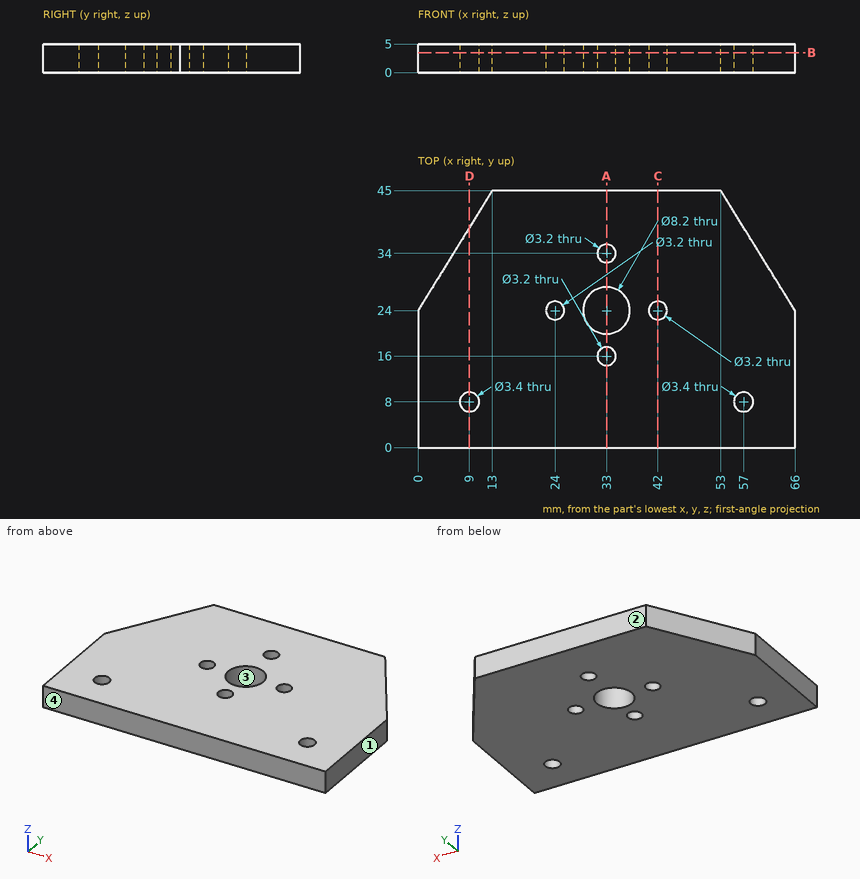
Study the drawing (mm; zero at the part's minimum x, y, z) and answer. Coordinates: 2 decimals unless noted, no trailing zeros. Loops run counter-clockwise (first coordinate to the right, second up) from the corner with the lowest first, then second, coordinate; pieces in that order, holes last. Notation, with made-up numbers: M 48.5,74.5 L 84.5,74.5 A24 cw 84.5,93.5 Z; hole C 60.5,-33 d3. An arc over 180 degrees is marked long. Answer as a JSON object with one key per item and string values. Group by question number.
Item 1: Section A-A (x = 33) is taken. Write down the section's boundary in (y, z).
Item 2: Section D-D (x = 9) is taken. Write down the section's boundary in (y, z).
Item 3: Section C-C (x = 42) is taken. Write down the section's boundary in (y, z).
Item 4: Consider L1, parallel to Y at x = 33, z = 3.55; L2, parallel to X at y = 26.5, z = 3.35; L3, parallel to X at y = 15.5, z = 2.7. Determine where each line is inside the solid, lowest interval first.
Item 5: Determine the mould class of the marked faces 1, 2, 3 and 4 for opening direction Y: +Y half, -Y half, draft (parallel to the pull), parting line (faces both ways), or undercut.
Item 6: Section B-B (z = 3.5) is taken. Write down the section's boundary in (x, y).
Item 7: Each of these flat-tipped pins is pushed along its axis until it touches: P1, Ø3, axis at y = 32.5, z = 3, coming from the +X side; P2, Ø1, axis at y = 37, z = 2, coming from the -X side; P3, Ø3, axis at x = 8, z = 4.5, coming from the +Y side. Where does it stop, or does it pass through?
Solved:
{
 "1": {"outline": "M 0,0 L 14.4,0 L 14.4,5 L 0,5 Z; M 17.6,0 L 19.9,0 L 19.9,5 L 17.6,5 Z; M 28.1,0 L 32.4,0 L 32.4,5 L 28.1,5 Z; M 35.6,0 L 45,0 L 45,5 L 35.6,5 Z"},
 "2": {"outline": "M 0,0 L 6.3,0 L 6.3,5 L 0,5 Z; M 9.7,0 L 38.54,0 L 38.54,5 L 9.7,5 Z"},
 "3": {"outline": "M 0,0 L 22.4,0 L 22.4,5 L 0,5 Z; M 25.6,0 L 45,0 L 45,5 L 25.6,5 Z"},
 "4": {"L1": "y = 0 to 14.4, 17.6 to 19.9, 28.1 to 32.4, 35.6 to 45", "L2": "x = 1.55 to 29.75, 36.25 to 64.45", "L3": "x = 0 to 31.48, 34.52 to 66"},
 "5": {"face 1": "draft", "face 2": "+Y half", "face 3": "undercut", "face 4": "-Y half"},
 "6": {"outline": "M 0,0 L 66,0 L 66,24 L 53,45 L 13,45 L 0,24 Z; hole C 9,8 d3.4; hole C 24,24 d3.2; hole C 33,24 d8.2; hole C 33,16 d3.2; hole C 33,34 d3.2; hole C 42,24 d3.2; hole C 57,8 d3.4"},
 "7": {"P1": "stops at x = 61.67", "P2": "stops at x = 7.74", "P3": "stops at y = 39.35"}
}
